from build123d import *

# Parameters (mm, degrees)
SKETCH1_W           = 15.875
SKETCH1_H           = 6.35
BOSS_EXTRUDE1_DEPTH = 6.35
FILLET1_R           = 2.54


with BuildPart() as part:
    # Sketch1 → Boss-Extrude1 (new body)
    with BuildSketch(Plane(origin=(0, 0, 0), x_dir=(0, 0, -1), z_dir=(1, 0, 0))):
        Polygon((-26.9875, 88.9), (-33.3375, 88.9), (-109.5375, -88.9), (-103.1875, -88.9), (-87.3125, -88.9), (-80.9625, -88.9), (-80.9625, -82.55), (4.7625, -82.55), (4.7625, -88.9), (11.1125, -88.9), (26.9875, -88.9), (33.3375, -88.9), (33.3375, 88.9), (26.9875, 88.9), (11.1125, 88.9), (-11.1125, 88.9), align=None)
        with Locations((19.05, -92.075)):
            Rectangle(SKETCH1_W, SKETCH1_H)
        with Locations((-19.05, 92.075)):
            Rectangle(SKETCH1_W, SKETCH1_H)
        with Locations((19.05, 92.075)):
            Rectangle(SKETCH1_W, SKETCH1_H)
        with Locations((-95.25, -92.075)):
            Rectangle(SKETCH1_W, SKETCH1_H)
    extrude(amount=BOSS_EXTRUDE1_DEPTH)

    # Fillet1
    fillet1_edges = [part.edges().sort_by_distance(p)[0] for p in [
        (3.175, -82.55, 80.9625),
        (3.175, -88.9, 80.9625),
        (3.175, -88.9, 109.5375),
        (3.175, 88.9, 33.3375),
        (3.175, 88.9, -33.3375),
        (3.175, -88.9, -33.3375),
        (3.175, -88.9, -4.7625),
        (3.175, -82.55, -4.7625),
    ]]
    fillet(fillet1_edges, radius=FILLET1_R)


solid = part.part
Check sheet for the modelled part. Datum: model origin and axes. Units: mm. A direction names the side the tool comes from. Give positions to 0.01 mm unless a question says otherwise; leave off trailing zeros. Order: outer loops, then holes, each group sorted by start corner. A loop starts at its lowest first (then second) coordinate and runs counter-clockwise, first axis right, second up. Notation, with made-up numbers: M 25,57.25 L 37,57.25 A27 cw 37,80.25 Z; hole C 23.25,49 d6. An arc over 180 degrees is marked long. Answer as CSV lines item,"result". Start each with the question number.
Item 1: Cross-section at B-B on z = 24. Enter the section's corners in (x, y), plus the area to 3 significant figures.
Item 2: Thickness scan on line 1 (Y direction, x = 1.25, z = 21); line 2 (Y direction, x = 4, z = -9); line 3 (Z direction, x = 3.25, y = -84). Record the ranges inside material, lowest first. Write a range as [from, to].
Item 3: Mould release check, pull along Z, two halves, no side actions. Record for faces 1 (the face through (3, -82.55, 39)), 2 (the face through (3, -92, -26.988)), 3 (the face through (3, 88.9, -29)): +Z half, -Z half, draft (parallel to the pull), parting line (faces both ways), or undercut.
Item 4: Cross-section at C-C on y = 27.5. Enter the section's corners in (x, z), plus the area to 3 significant figures.
Item 5: Gauge pin test, flat ends, axial feed: P1, Ø1.2, axis at x = 2.5, z = 104.5, coming from the -Y side; P2, Ø3, axis at x = 4.5, y = -92.5, coming from the -Z side; P3, Ø3, axis at y = 60.5, z = -3.5, coming from the -X side; P4, Ø1.9, axis at x = 3.5, z = -28, coming from the +Y side. Record the tip position at first contact, or that the pin passes through.
Item 6: Tool access check on faces 4 (the face through (3, -88.9, 85)), 5 (the face through (3, 92, -26.988)), 6 (the face through (3, 88.9, 29)), 7 (the face through (3, -88.9, -29)). Record the directions out of +Z, -Z, +X, -X, +Y, -Y that give a thin tool (end or side, any length) a straight path to the whole face; none if there is none.
Established:
1,outline,"M 0,-82.55 L 6.35,-82.55 L 6.35,95.25 L 0,95.25 Z"
1,area,"1,130 mm^2"
2,line 1,"y = [-82.55, 95.25]"
2,line 2,"y = [-88.9, 88.9]"
2,line 3,"z = [-33.34, -4.52], [80.72, 107.44]"
3,face 1,"undercut"
3,face 2,"-Z half"
3,face 3,"draft"
4,outline,"M 0,-33.34 L 6.35,-33.34 L 6.35,59.65 L 0,59.65 Z"
4,area,"590 mm^2"
5,P1,"stops at y = -88.9"
5,P2,"stops at z = -26.99"
5,P3,"stops at x = 0"
5,P4,"stops at y = 88.9"
6,face 4,"+X, -X, -Y"
6,face 5,"-Z, +X, -X, +Y"
6,face 6,"+Z, +X, -X, +Y"
6,face 7,"-Z, +X, -X, -Y"
